Geometry check sheet. Reference: the model listing, model coordinates, mm. A direction names the side the tool comes from. Round coordinates to 2 decimals unless told otherwise and drop trailing zeros. Loops run counter-clockwise (first coordinate to the right, second up) from the corner with the lowest first, then second, coordinate; pieces in that order, holes last. Notation, with made-up numbers: M 45,25.25 L 72,25.25 A23 cw 72,46.25 Z; hole C 30.5,39.25 d4. An arc over 180 degrees is marked long. Write item = value, one per line.
from build123d import *

# Parameters (mm, degrees)
F0_W     = 34.5
F0_H     = 6
F0_R     = 1.4
F1_DEPTH = 13
F2_R     = 1.4
F3_DEPTH = 10
F4_R     = 1.4
F5_DEPTH = 10


with BuildPart() as f1:
    # F0 (on Top) → F1 (new body)
    with BuildSketch(Plane.XY):
        with Locations((17.25, 3)):
            Rectangle(F0_W, F0_H)
        with Locations((9, 3)):
            Circle(F0_R, mode=Mode.SUBTRACT)
        with Locations((25.5, 3)):
            Circle(F0_R, mode=Mode.SUBTRACT)
    extrude(amount=F1_DEPTH)

    # F2 (on face) → F3 (cut)
    with BuildSketch(Plane(origin=(0, 0, 0), x_dir=(0, -1, 0), z_dir=(-1, 0, 0))):
        with Locations((-3, 8.5)):
            Circle(F2_R)
    extrude(amount=-F3_DEPTH, mode=Mode.SUBTRACT)

    # F4 (on face) → F5 (cut)
    with BuildSketch(Plane.YZ.offset(34.5)):
        with Locations((3, 8.5)):
            Circle(F4_R)
    extrude(amount=-F5_DEPTH, mode=Mode.SUBTRACT)


solid = f1.part
(1) Tool access check on faces 5 (the cylindrical face through (24.9, 1.6, 8.5)), 6 (the flat face through (34.5, 3, 6)), 7 (the cylindrical face through (4.44, 1.71, 7.96)). Record the directions out of +Z, -Z, +X, -X, +Y, -Y that give a thin tool (end or side, any length) a straight path to the whole face; none if there is none.
Result set:
face_5 = +X
face_6 = +Z, -Z, +X, +Y, -Y
face_7 = -X
(2) Sectioned sample at B-B on y = 3. Record the cut outline in (x, z).
Result set:
outline = M 0,0 L 7.6,0 L 7.6,7.1 L 0,7.1 Z; M 0,9.9 L 7.6,9.9 L 7.6,13 L 0,13 Z; M 10.4,0 L 24.1,0 L 24.1,13 L 10.4,13 Z; M 26.9,0 L 34.5,0 L 34.5,7.1 L 26.9,7.1 Z; M 26.9,9.9 L 34.5,9.9 L 34.5,13 L 26.9,13 Z
(3) Sectioned sample at C-C on z = 12. Record the cut outline in (x, y), then the cut area to 3 significant figures.
Result set:
outline = M 0,0 L 34.5,0 L 34.5,6 L 0,6 Z; hole C 9,3 d2.8; hole C 25.5,3 d2.8
area = 195 mm2
(4) Sectioned sample at A-A on x = 29. Record the cut outline in (y, z), then the cut area to 3 significant figures.
Result set:
outline = M 0,0 L 6,0 L 6,13 L 0,13 Z; hole C 3,8.5 d2.8
area = 71.8 mm2
(5) Material ranges on line 1 along Y through (x, z) = (8, 1); line 2 along Y through (x, z) = (31.5, 8.5); line 3 along Z through (x, y) = (4.5, 3), recorded low to high. Write a range as from..to.
Result set:
line_1 = 0..2.02, 3.98..6
line_2 = 0..1.6, 4.4..6
line_3 = 0..7.1, 9.9..13
(6) Depth check by flat-ended pin: pin 1 Ø2.5 at (y, z) = (3, 8.5) entering from +X. Enter the tip coordinate at first touch or a pass-through.
Result set:
pin_1 = 24.5
(7) Sectioned sample at D-D on z = 9. Record the cut outline in (x, y), then the cut area to 3 significant figures.
Result set:
outline = M 0,0 L 34.5,0 L 34.5,1.69 L 26,1.69 A1.4 cw 25,1.69 L 24.5,1.69 L 24.5,2.02 A1.4 cw 24.5,3.98 L 24.5,4.31 L 25,4.31 A1.4 cw 26,4.31 L 34.5,4.31 L 34.5,6 L 0,6 L 0,4.31 L 8.5,4.31 A1.4 cw 9.5,4.31 L 10,4.31 L 10,3.98 A1.4 cw 10,2.02 L 10,1.69 L 9.5,1.69 A1.4 cw 8.5,1.69 L 0,1.69 Z
area = 153 mm2
(8) Release check for a two-part mould opening along Z. For faces 1 (the flat face through (17, 3, 0)), 2 (the cylindrical face through (24.9, 4.4, 8.5)), 3 (the flat face through (17, 3, 13)), 4 (the flat face through (17, 0, 6)) record: released by +Z, released by -Z, zero draft, split by the parting line, or undercut.
Result set:
face_1 = released by -Z
face_2 = undercut
face_3 = released by +Z
face_4 = zero draft
